Could you check a few things on this model? Use its own coordinates, in mm. Face numbers are marked on the shaded views. Give positions to 0.01 mm unless a question says otherwise; leave off trailing zeros. Loops run counter-clockwise (first coordinate to the right, second up) from the corner with the lowest first, then second, coordinate; pieces in that order, holes last. Notation, with made-up numbers: (10.25, 15) - (53.25, 15) arc R23 ccw to (53.25, 33) - close; hole circle Ø10 at (78, 29). An arc over 180 degrees is marked (long way). One line per item, written item: value. Start each with the question number.
Q1. If I drill on line 1 (X direction, y = 135, z = -1); line 2 (Z direction, x = 137.5, y = 271); line 3 (Y direction, x = 332, z = -46.5), over which ranges is the centre line in solid material (lowest first)? Write a range as from..to.
Q2. I want a section at D-D (z = -52). Please give me the cut outline in (x, y).
Q3. If we mould it in two halves opening along Y, with no side actions, what happens to the marked faces 1, 2, 3 and 4? For each: released by +Y, released by -Y, zero draft, split by the parting line, or undercut.
Q4. I'm going to push flat-ended pins straight in: P1, Ø3, axis at x = 492.5, y = 140.5, coming from the +Z side; P2, Ø11, axis at y = -46, z = 3, coming from the -X side; P3, Ø2, axis at x = 276.5, y = 277, coming from the -Z side. Where does each tip first touch, or does it pass through?
Q5. I want a section at A-A (x = 199.5). Please give me the cut outline in (y, z).
Q6. I want a section at B-B (y = 173.5). Please give me the cut outline in (x, z).
Q7. I want a section at C-C (x = 408.5). Please give me the cut outline in (y, z).
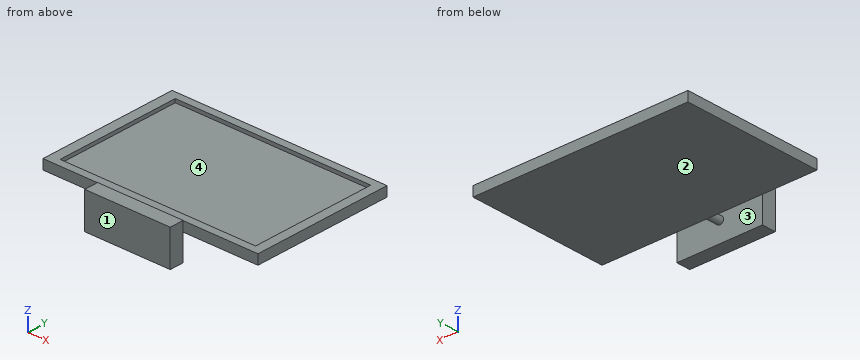
```python
from build123d import *

# Parameters (mm, degrees)
CROQUIS1_W              = 24.727272727
CROQUIS1_H              = 360
SALIENTE_EXTRUIR1_DEPTH = 549
CROQUIS3_W              = 499.313479992
CROQUIS3_H              = 321.141187852
CORTAR_EXTRUIR1_DEPTH   = 9
CROQUIS4_R              = 9.403689311
SALIENTE_EXTRUIR2_DEPTH = 36
CROQUIS5_W              = 218.404745205
CROQUIS5_H              = 91.241456057
SALIENTE_EXTRUIR3_DEPTH = 36


with BuildPart() as part:
    # Croquis1 → Saliente-Extruir1 (new body)
    with BuildSketch(Plane(origin=(0, 0, 0), x_dir=(0, 0, -1), z_dir=(1, 0, 0))):
        with Locations((12.363636364, 180)):
            Rectangle(CROQUIS1_W, CROQUIS1_H)
    extrude(amount=SALIENTE_EXTRUIR1_DEPTH)

    # Croquis3 → Cortar-Extruir1 (cut)
    with BuildSketch(Plane.XY):
        with Locations((275.577654993, 180)):
            Rectangle(CROQUIS3_W, CROQUIS3_H)
    extrude(amount=-CORTAR_EXTRUIR1_DEPTH, mode=Mode.SUBTRACT)

    # Croquis4 → Saliente-Extruir2 (add)
    with BuildSketch(Plane.XZ):
        with Locations((280.998241646, -13.903750832)):
            Circle(CROQUIS4_R)
    extrude(amount=SALIENTE_EXTRUIR2_DEPTH)

    # Croquis5 → Saliente-Extruir3 (add)
    with BuildSketch(Plane.XZ.offset(36)):
        with Locations((281.684366619, -18.111129658)):
            Rectangle(CROQUIS5_W, CROQUIS5_H)
    extrude(amount=SALIENTE_EXTRUIR3_DEPTH)


solid = part.part
```
Worked answers:
1. line 1: x = 0..25.92, 525.23..549
1. line 2: z = -24.73..-9
1. line 3: y = -72..-36
2. outline: (172.48, -72) - (390.89, -72) - (390.89, -36) - (172.48, -36) - close
3. face 1: released by -Y
3. face 2: zero draft
3. face 3: undercut
3. face 4: undercut
4. P1: stops at z = -9
4. P2: stops at x = 172.48
4. P3: stops at z = -24.73
5. outline: (-72, -63.73) - (-36, -63.73) - (-36, 27.51) - (-72, 27.51) - close; (0, -24.73) - (360, -24.73) - (360, 0) - (340.57, 0) - (340.57, -9) - (19.43, -9) - (19.43, 0) - (0, 0) - close
6. outline: (0, -24.73) - (549, -24.73) - (549, 0) - (525.23, 0) - (525.23, -9) - (25.92, -9) - (25.92, 0) - (0, 0) - close
7. outline: (0, -24.73) - (360, -24.73) - (360, 0) - (340.57, 0) - (340.57, -9) - (19.43, -9) - (19.43, 0) - (0, 0) - close
